```python
from build123d import *

# Parameters (mm, degrees)
F0_W     = 180
F0_H     = 35
F1_DEPTH = 27
F3_DEPTH = 15
F4_SIZE  = 1
F5_R     = 2
F6_DEPTH = 30


with BuildPart() as f1:
    # F0 (on Front) → F1 (new body)
    with BuildSketch(Plane.XZ):
        Rectangle(F0_W, F0_H)
    extrude(amount=F1_DEPTH)

    # F2 (on face) → F3 (cut)
    with BuildSketch(Plane(origin=(0, 0, 0), x_dir=(-1, 0, 0), z_dir=(0, 1, 0))):
        with BuildLine():
            Line((32, 12.5), (-77, 12.5))
            ThreePointArc((-77, 12.5), (-79.12132, 11.62132), (-80, 9.5))
            Line((-80, 9.5), (-80, -3.5))
            ThreePointArc((-80, -3.5), (-79.12132, -5.62132), (-77, -6.5))
            Line((-77, -6.5), (32, -6.5))
            ThreePointArc((32, -6.5), (34.12132, -5.62132), (35, -3.5))
            Line((35, -3.5), (35, 9.5))
            ThreePointArc((35, 9.5), (34.12132, 11.62132), (32, 12.5))
        make_face()
    extrude(amount=-F3_DEPTH, mode=Mode.SUBTRACT)

    # F4
    f4_edges = [f1.edges().sort_by_distance(p)[0] for p in [
        (-90, -13.5, -17.5),
        (-90, -13.5, 17.5),
        (90, -13.5, -17.5),
        (90, -13.5, 17.5),
        (0, 0, 17.5),
        (0, 0, -17.5),
        (90, -27, 0),
        (90, 0, 0),
        (-90, 0, 0),
        (-90, -27, 0),
        (0, -27, -17.5),
        (0, -27, 17.5),
    ]]
    chamfer(f4_edges, length=F4_SIZE)

    # F5 (on face) → F6 (cut)
    with BuildSketch(Plane.XY.offset(17.5)):
        with Locations((-80, -21)):
            Circle(F5_R)
        with Locations((10, -21)):
            Circle(F5_R)
    extrude(amount=-F6_DEPTH, mode=Mode.SUBTRACT)


solid = f1.part
```
Model file for the job. Use its own axes, mm. A direction names the side the tool comes from. Coordinates: 2 decimals unless noted, no trailing zeros. Loops run counter-clockwise (first coordinate to the right, second up) from the corner with the lowest first, then second, coordinate; pieces in that order, holes last. Notation, with made-up numbers: (76, 56) -> (115, 56) arc R20 cw to (115, 67) -> close; hole circle Ø10 at (81, -23). An arc over 180 degrees is marked (long way). Answer as a JSON object with one key per item and string values.
Q1. Cut at B-B (y = -10.5). List the corners of the cut face in (x, z).
Report:
{"outline": "(-90, -16.5) -> (-89, -17.5) -> (89, -17.5) -> (90, -16.5) -> (90, 16.5) -> (89, 17.5) -> (-89, 17.5) -> (-90, 16.5) -> close; hole (-35, -3.5) arc R3 ccw to (-32, -6.5) -> (77, -6.5) arc R3 ccw to (80, -3.5) -> (80, 9.5) arc R3 ccw to (77, 12.5) -> (-32, 12.5) arc R3 ccw to (-35, 9.5) -> close"}
Q2. Cut at C-C (x = 33). List the corners of the cut face in (y, z), and give its area (3 significant figures).
Report:
{"outline": "(-27, -16.5) -> (-26, -17.5) -> (-1, -17.5) -> (0, -16.5) -> (0, -6.5) -> (-15, -6.5) -> (-15, 12.5) -> (0, 12.5) -> (0, 16.5) -> (-1, 17.5) -> (-26, 17.5) -> (-27, 16.5) -> close", "area": "658 mm2"}
Q3. Probe probe 1 along Y at (x, z) = (10, 6); probe 2 along Z at (x, y) = (11, -9.25); probe 3 along Y at (x, z) = (-80, -6). List the from-to ranges inside material, lowest first.
Report:
{"probe 1": "y = -27 to -23, -19 to -15", "probe 2": "z = -17.5 to -6.5, 12.5 to 17.5", "probe 3": "y = -27 to -23, -19 to 0"}
Q4. Cut at A-A (z = 0). List the corners of the cut face in (x, y).
Report:
{"outline": "(-90, -26) -> (-89, -27) -> (89, -27) -> (90, -26) -> (90, -1) -> (89, 0) -> (80, 0) -> (80, -15) -> (-35, -15) -> (-35, 0) -> (-89, 0) -> (-90, -1) -> close; hole circle Ø4 at (-80, -21); hole circle Ø4 at (10, -21)"}
Q5. 3-axis set-ups, long thin cutter, end or side, ignore diameter. For faces 4 (the cylindrical face through (-78.092, -20.399, 2.71)), 5 (the cylindrical face through (79.1, -7.4, 11.64)), 6 (the flat face through (-1, -13, -17.5)): which of +Z, -Z, +X, -X, +Y, -Y reach the whole face in a straight line?
Report:
{"face 4": "+Z", "face 5": "+Y", "face 6": "-Z, +X, -X, +Y, -Y"}
Q6. Cut at D-D (y = -21). List the corners of the cut face in (x, z).
Report:
{"outline": "(-90, -16.5) -> (-89, -17.5) -> (89, -17.5) -> (90, -16.5) -> (90, 16.5) -> (89, 17.5) -> (12, 17.5) -> (12, -12.5) -> (8, -12.5) -> (8, 17.5) -> (-78, 17.5) -> (-78, -12.5) -> (-82, -12.5) -> (-82, 17.5) -> (-89, 17.5) -> (-90, 16.5) -> close"}
Q7. Pull direction Z, two halves, no side cores. Call faces 1 (the flat face through (-80, -21, -12.5)), 2 (the flat face through (22, -7, 12.5)), 3 (the flat face through (90, -13, 0)): released by +Z, released by -Z, zero draft, split by the parting line, or undercut.
Report:
{"face 1": "released by +Z", "face 2": "undercut", "face 3": "zero draft"}
Q8. Flat gauge pins, fed straight in: P1, Ø3.5, axis at x = 10, y = -21, coming from the +Z side; P2, Ø6, axis at x = 65, z = 2, coming from the +Y side; P3, Ø5, axis at x = -80, y = -21, coming from the +Z side. Where does each tip first touch, or does it go through?
Report:
{"P1": "stops at z = -12.5", "P2": "stops at y = -15", "P3": "stops at z = 17.5"}
